```python
from build123d import *

# Parameters (mm, degrees)
BOSS_EXTRUDE1_DEPTH = 3
SKETCH2_R           = 2.5
CUT_EXTRUDE1_DEPTH  = 3


with BuildPart() as part:
    # Sketch1 → Boss-Extrude1 (new body)
    with BuildSketch(Plane.XY):
        with BuildLine():
            Line((1.5, 60), (19.378679656, 60))
            ThreePointArc((19.378679656, 60), (19.952704805, 59.885819299), (20.439339828, 59.560660172))
            Line((20.439339828, 59.560660172), (59.560660172, 20.439339828))
            ThreePointArc((59.560660172, 20.439339828), (59.885819299, 19.952704805), (60, 19.378679656))
            Line((60, 19.378679656), (60, 1.5))
            ThreePointArc((60, 1.5), (59.560660172, 0.439339828), (58.5, 0))
            Line((58.5, 0), (1.5, 0))
            ThreePointArc((1.5, 0), (0.439339828, 0.439339828), (0, 1.5))
            Line((0, 1.5), (0, 58.5))
            ThreePointArc((0, 58.5), (0.439339828, 59.560660172), (1.5, 60))
        make_face()
    extrude(amount=-BOSS_EXTRUDE1_DEPTH)

    # Sketch2 → Cut-Extrude1 (cut)
    with BuildSketch(Plane.XY):
        with Locations((10, 10)):
            Circle(SKETCH2_R)
        with Locations((30, 10)):
            Circle(SKETCH2_R)
        with Locations((50, 10)):
            Circle(SKETCH2_R)
        with Locations((10, 30)):
            Circle(SKETCH2_R)
        with Locations((10, 50)):
            Circle(SKETCH2_R)
    extrude(amount=-CUT_EXTRUDE1_DEPTH, mode=Mode.SUBTRACT)


solid = part.part
```
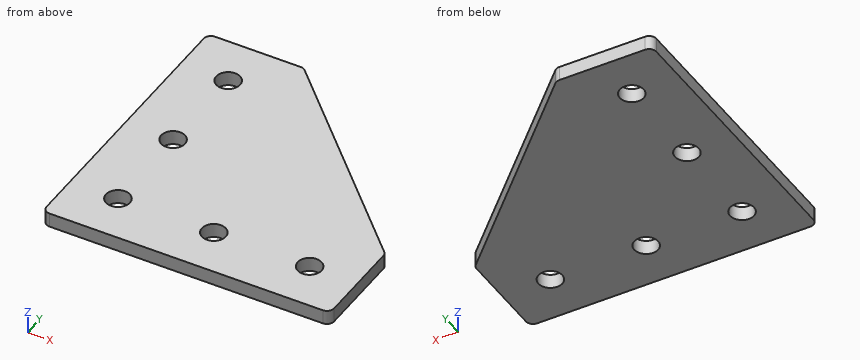
Design review of the part built by this model. Coordinates are the model's own, in mm. Coordinates: 2 decimals unless noted, no trailing zeros. Loops run counter-clockwise (first coordinate to the right, second up) from the corner with the lowest first, then second, coordinate; pieces in that order, holes last. Notation, with made-up numbers: M 10.25,68 L 19.25,68 A18 cw 19.25,91 Z; hole C 54.5,74.25 d1. An arc over 180 degrees is marked long. One line per question, with ' | ' between items.
(1) We need section C-C (x = 50). Give the boundary of the cut face in (y, z), and give its area (3 significant figures).
Filled in:
outline: M 0,-3 L 7.5,-3 L 7.5,0 L 0,0 Z; M 12.5,-3 L 30,-3 L 30,0 L 12.5,0 Z | area: 75.0 mm^2
(2) We need section D-D (y = 30). Give the boundary of the cut face in (x, z).
Filled in:
outline: M 0,-3 L 7.5,-3 L 7.5,0 L 0,0 Z; M 12.5,-3 L 50,-3 L 50,0 L 12.5,0 Z
(3) We need section A-A (y = 10). Give the boundary of the cut face in (x, z).
Filled in:
outline: M 0,-3 L 7.5,-3 L 7.5,0 L 0,0 Z; M 12.5,-3 L 27.5,-3 L 27.5,0 L 12.5,0 Z; M 32.5,-3 L 47.5,-3 L 47.5,0 L 32.5,0 Z; M 52.5,-3 L 60,-3 L 60,0 L 52.5,0 Z
(4) For pin 1 Ø1.5 at (x, z) = (22, -2) entering from +Y; pin 2 Ø3 at (x, y) = (10, 10) entering from +Z, all flat-tipped, find the tip position at first contact; note any pin that passes through.
Filled in:
pin 1: stops at y = 58.75 | pin 2: passes through
(5) Wall thickness on probe 1 along Y at (x, z) = (10, -2.4); probe 2 along Y at (x, z) = (8, -0.15); probe 3 along Y at (x, z) = (51, -2.5): over which ranges is each line inside the solid? List them lowest first.
Filled in:
probe 1: y = 0 to 7.5, 12.5 to 27.5, 32.5 to 47.5, 52.5 to 60 | probe 2: y = 0 to 8.5, 11.5 to 28.5, 31.5 to 48.5, 51.5 to 60 | probe 3: y = 0 to 7.71, 12.29 to 29
